from build123d import *

# Parameters (mm, degrees)
F1_DEPTH        = 14.224
F2_DEPTH        = 5.715
F3_D            = 12.7
F3_COPIES_COUNT = 4
F5_R            = 34.29
F6_DEPTH        = 12.7
F6_TAPER        = 5
F7_D            = 49.022
F7_DEPTH        = 14.225
F8_D            = 49.022


# Not quite as in the source:
# - a pattern or mirror of a feature is missing from the dataset's text; its kind, count and spacing are read off the source's solid


with BuildPart() as f1:
    # F0 (on Top) → F1 (new body)
    with BuildSketch(Plane.XY):
        with BuildLine():
            Line((35.0229988722, 47.625), (-35.0229988722, 47.625))
            ThreePointArc((-35.0229988722, 47.625), (-43.9339593262, 43.9339593262), (-47.625, 35.0229988722))
            Line((-47.625, 35.0229988722), (-47.625, -35.0229988722))
            ThreePointArc((-47.625, -35.0229988722), (-43.9339593262, -43.9339593262), (-35.0229988722, -47.625))
            Line((-35.0229988722, -47.625), (35.0229988722, -47.625))
            ThreePointArc((35.0229988722, -47.625), (43.9339593262, -43.9339593262), (47.625, -35.0229988722))
            Line((47.625, -35.0229988722), (47.625, 35.0229988722))
            ThreePointArc((47.625, 35.0229988722), (43.9339593262, 43.9339593262), (35.0229988722, 47.625))
        make_face()
        with BuildLine():
            Line((22.3801912029, -40.005), (-22.3801912029, -40.005))
            ThreePointArc((-22.3801912029, -40.005), (-25.4141248226, -25.4141248226), (-40.005, -22.3801912029))
            Line((-40.005, -22.3801912029), (-40.005, 22.3801912029))
            ThreePointArc((-40.005, 22.3801912029), (-25.4141248226, 25.4141248226), (-22.3801912029, 40.005))
            Line((-22.3801912029, 40.005), (22.3801912029, 40.005))
            ThreePointArc((22.3801912029, 40.005), (25.4141248226, 25.4141248226), (40.005, 22.3801912029))
            Line((40.005, 22.3801912029), (40.005, -22.3801912029))
            ThreePointArc((40.005, -22.3801912029), (25.4141248226, -25.4141248226), (22.3801912029, -40.005))
        make_face(mode=Mode.SUBTRACT)
        with BuildLine():
            ThreePointArc((-40.005, -22.3801912029), (-25.4141248226, -25.4141248226), (-22.3801912029, -40.005))
            Line((-22.3801912029, -40.005), (22.3801912029, -40.005))
            ThreePointArc((22.3801912029, -40.005), (25.4141248226, -25.4141248226), (40.005, -22.3801912029))
            Line((40.005, -22.3801912029), (40.005, 22.3801912029))
            ThreePointArc((40.005, 22.3801912029), (25.4141248226, 25.4141248226), (22.3801912029, 40.005))
            Line((22.3801912029, 40.005), (-22.3801912029, 40.005))
            ThreePointArc((-22.3801912029, 40.005), (-25.4141248226, 25.4141248226), (-40.005, 22.3801912029))
            Line((-40.005, 22.3801912029), (-40.005, -22.3801912029))
        make_face()
    extrude(amount=F1_DEPTH)

    # F0 (on Top) → F2 (cut)
    with BuildSketch(Plane.XY):
        with BuildLine():
            ThreePointArc((-40.005, -22.3801912029), (-25.4141248226, -25.4141248226), (-22.3801912029, -40.005))
            Line((-22.3801912029, -40.005), (22.3801912029, -40.005))
            ThreePointArc((22.3801912029, -40.005), (25.4141248226, -25.4141248226), (40.005, -22.3801912029))
            Line((40.005, -22.3801912029), (40.005, 22.3801912029))
            ThreePointArc((40.005, 22.3801912029), (25.4141248226, 25.4141248226), (22.3801912029, 40.005))
            Line((22.3801912029, 40.005), (-22.3801912029, 40.005))
            ThreePointArc((-22.3801912029, 40.005), (-25.4141248226, 25.4141248226), (-40.005, 22.3801912029))
            Line((-40.005, 22.3801912029), (-40.005, -22.3801912029))
        make_face()
    extrude(amount=F2_DEPTH, mode=Mode.SUBTRACT)

    # F3 (through all)
    with Locations(Plane(origin=(0, 0, 0), x_dir=(1, 0, 0), z_dir=(0, 0, -1))):
        with Locations((-35.0229988722, -35.0229988722)):
            f3 = Hole(F3_D / 2)

    # F3_copies: F3 ×4 about axis
    f3_copies_axis = Axis((0, 0, 0), (0, 0, 1))
    for i in range(1, F3_COPIES_COUNT):
        add(f3.rotate(f3_copies_axis, i * 360 / F3_COPIES_COUNT), mode=Mode.SUBTRACT)

    # F5 (on face) → F6 (join)
    with BuildSketch(Plane.XY.offset(14.224)):
        Circle(F5_R)
    extrude(amount=F6_DEPTH, taper=F6_TAPER)

    # F7 (through all, one way)
    with BuildSketch(Plane.XY.offset(14.224)):
        with Locations((0, 0)):
            Circle(F7_D / 2)
    extrude(amount=-F7_DEPTH, mode=Mode.SUBTRACT)

    # F8 (through all)
    with Locations(Plane(origin=(0, 0, 14.224), x_dir=(1, 0, 0), z_dir=(0, 0, -1))):
        with Locations((0, 0)):
            Hole(F8_D / 2)


solid = f1.part
The model under review builds one solid part; all positions refer to its coordinate system, in mm. A direction names the side the tool comes from. Coordinates: 2 decimals unless noted, no trailing zeros. Write each loop counter-clockwise with the first axis right and the second up, starting at its lowest first coordinate (ties: lowest second). Pieces come first, ordered by that corner, then holes. Notation, with made-up numbers: M 50.5,-18 L 56.5,-18 A17 ccw 56.5,1 Z; hole C 86,70 d8. An arc over 180 degrees is marked long. Put each result on its own line as item: value.
1) Clearance check with flat-ended pins moving along their axes: pin 1 Ø1 at (x, y) = (-13.5, -28) entering from -Z (3 decimals); pin 2 Ø1.5 at (x, y) = (30.5, -19) entering from +Z; pin 3 Ø14.5 at (x, y) = (-35.02, -35.02) entering from -Z; pin 4 Ø6 at (x, z) = (33.5, 20) entering from -Y. State where each tip first meets the part, or that it passes through.
Computed:
pin 1: stops at z = 5.715
pin 2: stops at z = 14.22
pin 3: stops at z = 0
pin 4: stops at y = -14.56
2) Add section B-B on z = 9. Give the boundary of the cut face in (x, y) (3 decimals), then the cut area to 3 significant figures.
Computed:
outline: M -47.625,-35.023 A12.602 ccw -35.023,-47.625 L 35.023,-47.625 A12.602 ccw 47.625,-35.023 L 47.625,35.023 A12.602 ccw 35.023,47.625 L -35.023,47.625 A12.602 ccw -47.625,35.023 Z; hole C -35.023,-35.023 d12.7; hole C -35.023,35.023 d12.7; hole C 0,0 d49.022; hole C 35.023,-35.023 d12.7; hole C 35.023,35.023 d12.7
area: 6,540 mm2
3) Add section C-C on x = 38.5. Give the boundary of the cut face in (y, z) (3 decimals), then the cut area to 3 significant figures.
Computed:
outline: M -47.136,0 L -40.336,0 L -40.336,14.224 L -47.136,14.224 Z; M -29.71,0 L -21.886,0 L -21.886,5.715 L 21.886,5.715 L 21.886,0 L 29.71,0 L 29.71,14.224 L -29.71,14.224 Z; M 40.336,0 L 47.136,0 L 47.136,14.224 L 40.336,14.224 Z
area: 788 mm2
4) Wall thickness on probe 1 along X at (y, z) = (11, 2.25) (3 decimals); probe 2 along Y at (x, z) = (-30, 2) (3 decimals); probe 3 along X at (y, z) = (38, 9.5): over which ranges is each line inside the solid? List them lowest first. Write a range as [from, to].
Computed:
probe 1: x = [-47.625, -40.005], [40.005, 47.625]
probe 2: y = [-47.625, -38.908], [-31.138, -22.396], [22.396, 31.138], [38.908, 47.625]
probe 3: x = [-47.27, -40.63], [-29.41, 29.41], [40.63, 47.27]
5) Draft analysis for pull direction Y (two halves, no side actions). For faces 4 (the flat face through (0, -47.625, 7)), 5 (the cylindrical face through (-25.26, 25.57, 2.82)), 6 (the flat face through (47.625, 0, 7)), 7 (the flat face through (-18, 18, 5.715)), state which applies: released by +Y, released by -Y, zero draft, split by the parting line, or undercut.
Computed:
face 4: released by -Y
face 5: undercut
face 6: zero draft
face 7: undercut
6) For faces 1 (the flat face through (0, 40.005, 3)), 2 (the flat face through (0, 47.625, 7)), 3 (the flat face through (-22, 32, 14.224)), list the 3-axis set-ups (+Z, -Z, +X, -X, +Y, -Y) from which the entire face can be reached by the end or side of a thin tool; tool diameter is ignored.
Computed:
face 1: -Z
face 2: +Z, -Z, +X, -X, +Y
face 3: +Z
7) Add section A-A on x = 0. Give the boundary of the cut face in (y, z) (3 decimals).
Computed:
outline: M -47.625,0 L -40.005,0 L -40.005,5.715 L -24.511,5.715 L -24.511,26.924 L -33.179,26.924 L -34.29,14.224 L -47.625,14.224 Z; M 24.511,5.715 L 40.005,5.715 L 40.005,0 L 47.625,0 L 47.625,14.224 L 34.29,14.224 L 33.179,26.924 L 24.511,26.924 Z
8) Add section D-D on z = 2.5. Give the boundary of the cut face in (x, y) (3 decimals), then the cut area to 3 significant figures.
Computed:
outline: M -47.625,-35.023 A12.602 ccw -35.023,-47.625 L 35.023,-47.625 A12.602 ccw 47.625,-35.023 L 47.625,35.023 A12.602 ccw 35.023,47.625 L -35.023,47.625 A12.602 ccw -47.625,35.023 Z; hole C -35.023,-35.023 d12.7; hole C -35.023,35.023 d12.7; hole M -40.005,-22.38 A13.589 cw -22.38,-40.005 L 22.38,-40.005 A13.589 cw 40.005,-22.38 L 40.005,22.38 A13.589 cw 22.38,40.005 L -22.38,40.005 A13.589 cw -40.005,22.38 Z; hole C 35.023,-35.023 d12.7; hole C 35.023,35.023 d12.7
area: 3,240 mm2
